Autodesk Inventor part; units mm, degrees
ref_plane "Start plane" through (0, 0, 0) normal (0, 0, 1) x (1, 0, 0)
ref_plane "End plane" through (0, 0, 112.5) normal (0, 0, 1) x (1, 0, 0)
ref_plane "YZ Plane" through (0, 0, 0) normal (1, 0, 0) x (0, 1, 0)
ref_plane "Start plane" through (0, 0, 0) normal (0, 0, 1) x (1, 0, 0)
ref_plane "End plane" through (0, 0, 112.5) normal (0, 0, 1) x (1, 0, 0)
sketch "Sketch" plane through (0, 0, 0) normal (0, 0, 1) x (1, 0, 0)
  line L0 (-9.525, -7.5438) -> (-9.525, 7.5438)
  line L1 (-7.5438, 9.525) -> (7.5438, 9.525)
  line L2 (9.525, 7.5438) -> (9.525, -7.5438)
  line L3 (7.5438, -9.525) -> (-7.5438, -9.525)
  arc A0 (-9.525, -7.5438) -> (-7.5438, -9.525) centre (-7.5438, -7.5438) ccw
  arc A1 (-7.5438, 9.525) -> (-9.525, 7.5438) centre (-7.5438, 7.5438) ccw
  arc A2 (9.525, 7.5438) -> (7.5438, 9.525) centre (7.5438, 7.5438) ccw
  arc A3 (7.5438, -9.525) -> (9.525, -7.5438) centre (7.5438, -7.5438) ccw
  arc A4 (-7.5438, 7.874) -> (-7.874, 7.5438) centre (-7.5438, 7.5438) ccw
  line L4 (-7.5438, 7.874) -> (7.5438, 7.874)
  arc A5 (7.874, 7.5438) -> (7.5438, 7.874) centre (7.5438, 7.5438) ccw
  line L5 (7.874, 7.5438) -> (7.874, -7.5438)
  arc A6 (7.5438, -7.874) -> (7.874, -7.5438) centre (7.5438, -7.5438) ccw
  line L6 (7.5438, -7.874) -> (-7.5438, -7.874)
  arc A7 (-7.874, -7.5438) -> (-7.5438, -7.874) centre (-7.5438, -7.5438) ccw
  line L7 (-7.874, -7.5438) -> (-7.874, 7.5438)
  line L8 (0, 13.9094) -> (0, -13.9094) construction
  line L9 (-13.9224, 0) -> (13.9871, 0) construction
  dimension "d10" = 19.05
  dimension "d11" = 19.05
  dimension "d12" = 1.651
  dimension "d15" = 9.525
  dimension "d16" = 9.525
  dimension "d17" = 1.9812
extrude "Body" add sketch "Sketch" along normal up to surface (112.5 mm away) from surface at 0
sketch "Sketch3" plane through (0, 0, 0) normal (0, 0, 1) x (1, 0, 0)
  line L0 (0, 0) -> (10, 0)
ref_plane "Work Plane3" through (0, 0, 0) normal (0, -1, 0) x (1, 0, 0)
sketch "Sketch4" plane through (0, 0, 0) normal (0, -1, 0) x (1, 0, 0)
  line L0 (-2, 0) -> (12, 0)
  line L1 (-2, 112.5) -> (12, 112.5)
  dimension "d19" = 112.5
ref_plane "Work Plane4" through (0, 7.5438, 0) normal (-1, 0, 0) x (0, 0, 1)
ref_plane "Work Plane5" through (7.5438, 0, 112.5) normal (0, 1, 0) x (1, 0, 0)
equation "\"d10\" = G_H"
equation "\"d11\" = G_W"
equation "\"d12\" = G_T"
equation "\"d15\" = 0.5 * d10"
equation "\"d16\" = 0.5 * d11"
equation "\"d17\" = G_IR"
equation "\"d3\" = G_L"
equation "\"G_W\" = 19.05"
equation "\"G_H\" = 19.05"
equation "\"G_T\" = 1.651"
equation "\"G_IR\" = 1.2 * G_T"
equation "\"G_L\" = d19"
equation "\"G_OFFSET_START\" = 0"
equation "\"G_OFFSET_END\" = 0"
equation "\"d14\" = G_OFFSET_END + B_L"
equation "\"B_L\" = 112.5"
properties part number "ASTM A513 - 3/4 x 3/4 x 13/200 - 4.4291339" material "Steel, Mild"
CAD build for the part. Positions are in the model's coordinates, mm. A direction names the side the tool comes from. Round coordinates to 2 decimals unless told otherwise and drop trailing zeros. Order: outer loops, then holes, each group sorted by start corner. A loop starts at its lowest first (then second) coordinate and runs counter-clockwise, first axis right, second up. Notation, with made-up numbers: (79, 80.25) - (107, 80.25) arc R14 ccw to (107, 98.25) - close; hole circle Ø7 at (-0.75, 18). An arc over 180 degrees is marked (long way). Use CSV: the item, a comma, the result in double quotes. Start each with the question number.
1) Wall check: L1, parallel to Y at x = -4, z = 30.5 (3 decimals); L2, parallel to X at y = 7.75, z = 23.5. Give the ranges that are in metal, low to high. Write a range as [from, to].
2) Pin check, flat tips, straight feed: pin 1 Ø5 at (x, y) = (-1, -7) entering from +Z; pin 2 Ø5 at (x, y) = (5, 0.5) entering from -Z. Stop position of each tip, or through.
3) Saw through at C-C (z = 34). List the corners of the cut face in (x, y) (3 decimals), and give its area (3 significant figures).
4) Two-plate mould, pull along X, no slides. Class faces 3 (the cylindrical face through (8.93, 8.96, 55.46)), 4 (the flat face through (0, 7.874, 55)), 5 (the flat face through (-9.525, 0, 55)): pulls with the +X half, pulls with the -X half, needs draft (parallel to the pull), parting line crosses it, or undercut.
5) Saw through at A-A (y = 3.75). List the corners of the cut face in (x, z) (3 decimals).
6) Tool access for faces 1 (the flat face through (7.874, 0, 55)), 2 (the flat face through (0, -9.525, 55)): list every direction of +Z, -Z, +X, -X, +Y, -Y with a clear straight run to the whole face (end or side of a thin tool).
Values follow:
1,L1,"y = [-9.525, -7.874], [7.874, 9.525]"
1,L2,"x = [-9.51, -7.8], [7.8, 9.51]"
2,pin 1,"stops at z = 112.5"
2,pin 2,"passes through"
3,outline,"(-9.525, -7.544) arc R1.981 ccw to (-7.544, -9.525) - (7.544, -9.525) arc R1.981 ccw to (9.525, -7.544) - (9.525, 7.544) arc R1.981 ccw to (7.544, 9.525) - (-7.544, 9.525) arc R1.981 ccw to (-9.525, 7.544) - close; hole (-7.874, -7.544) arc R0.33 ccw to (-7.544, -7.874) - (7.544, -7.874) arc R0.33 ccw to (7.874, -7.544) - (7.874, 7.544) arc R0.33 ccw to (7.544, 7.874) - (-7.544, 7.874) arc R0.33 ccw to (-7.874, 7.544) - close"
3,area,"112 mm2"
4,face 3,"pulls with the +X half"
4,face 4,"undercut"
4,face 5,"pulls with the -X half"
5,outline,"(-9.525, 0) - (-7.874, 0) - (-7.874, 112.5) - (-9.525, 112.5) - close; (7.874, 0) - (9.525, 0) - (9.525, 112.5) - (7.874, 112.5) - close"
6,face 1,"+Z, -Z"
6,face 2,"+Z, -Z, +X, -X, -Y"
